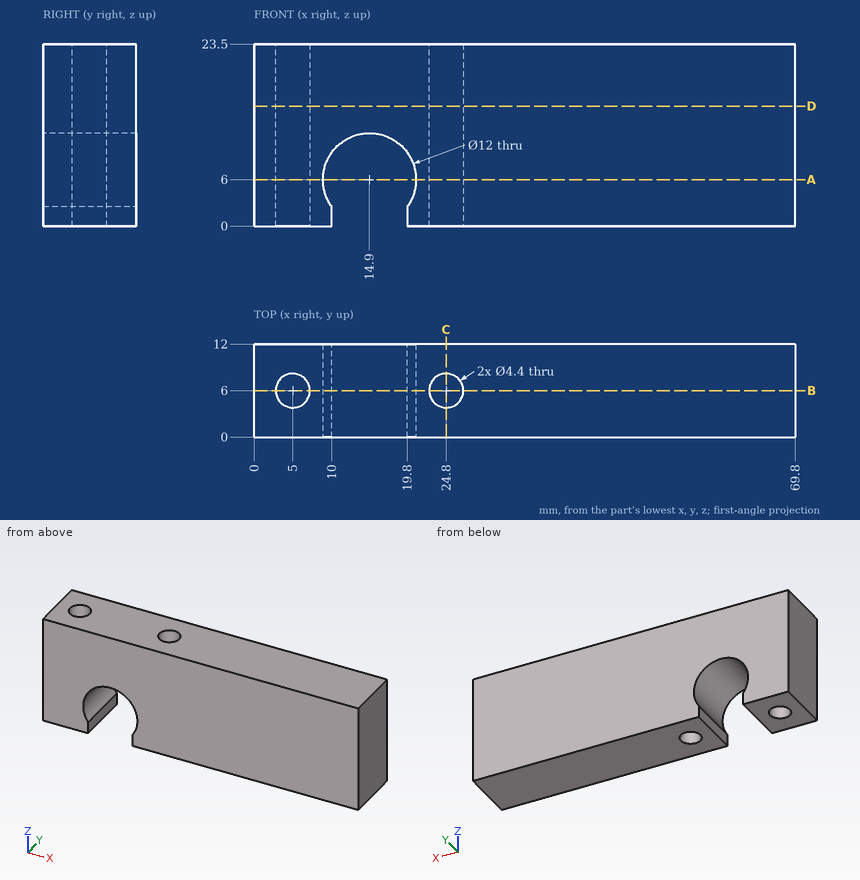
Print and shaded views of the part. All mm, measured from the part's lowest x, y and z. Coordinates: 2 decimals unless noted, no trailing zeros. Loops run counter-clockwise (first coordinate to the right, second up) from the corner with the lowest first, then second, coordinate; pieces in that order, holes last. Notation, with made-up numbers: (32.5, 5.5) -> (47.5, 5.5) arc R22 cw to (47.5, 16.5) -> close; hole circle Ø4 at (-13, -6.75). An arc over 180 degrees is marked (long way). Use one line per item in the form item = value. Start each with the question number.
(1) Cut at B-B on y = 6. Give the cut face in (x, z), and give its area (3 significant figures).
(2) Cut at D-D on z = 15.5. Give the cut face in (x, y), and give its area (3 significant figures).
(3) Cut at C-C on x = 24.8. Give the cut face in (y, z).
(4) Cut at A-A on z = 6. Give the cut face in (x, y), and give its area (3 significant figures).
(5) Flat gauge pins, fed straight in: pin 1 (7 mm diameter, centred on x = 14.9, z = 6, fed in from -Y); pin 2 (3 mm diameter, centred on x = 13.5, y = 9, fed in from -Z). Where does each tip first touch, or does it go through?
(6) Probe probe 1 along X at (y, z) = (9, 6); probe 2 along X at (y, z) = (4, 10.75); probe 3 along X at (y, z) = (5, 6). List the from-to ranges inside material, lowest first. Write a range as from..to.
Values:
q1.outline = (0, 0) -> (2.8, 0) -> (2.8, 23.5) -> (0, 23.5) -> close; (7.2, 0) -> (10, 0) -> (10, 2.54) arc R6 cw (long way) to (19.8, 2.54) -> (19.8, 0) -> (22.6, 0) -> (22.6, 23.5) -> (7.2, 23.5) -> close; (27, 0) -> (69.8, 0) -> (69.8, 23.5) -> (27, 23.5) -> close
q1.area = 1,310 mm2
q2.outline = (0, 0) -> (69.8, 0) -> (69.8, 12) -> (0, 12) -> close; hole circle Ø4.4 at (5, 6); hole circle Ø4.4 at (24.8, 6)
q2.area = 807 mm2
q3.outline = (0, 0) -> (3.8, 0) -> (3.8, 23.5) -> (0, 23.5) -> close; (8.2, 0) -> (12, 0) -> (12, 23.5) -> (8.2, 23.5) -> close
q4.outline = (0, 0) -> (8.9, 0) -> (8.9, 12) -> (0, 12) -> close; (20.9, 0) -> (69.8, 0) -> (69.8, 12) -> (20.9, 12) -> close; hole circle Ø4.4 at (5, 6); hole circle Ø4.4 at (24.8, 6)
q4.area = 663 mm2
q5.pin_1 = through
q5.pin_2 = 11.25
q6.probe_1 = 0..8.9, 20.9..69.8
q6.probe_2 = 0..4.08, 5.92..11.23, 18.57..23.88, 25.72..69.8
q6.probe_3 = 0..3.04, 6.96..8.9, 20.9..22.84, 26.76..69.8
